from build123d import *

# Parameters (mm, degrees)
BOSS_EXTRUDE1_DEPTH = 12.7
SKETCH2_W           = 4.3815
SKETCH2_H           = 12.607430492
CUT_EXTRUDE1_DEPTH  = 496.623170669
SKETCH3_R           = 5.08
BOSS_EXTRUDE2_DEPTH = 12.7


with BuildPart() as part:
    # Sketch1 → Boss-Extrude1 (new body)
    with BuildSketch(Plane.XY):
        Polygon((0, 0), (0, 6.35), (4.3815, 12.607430492), (5.1435, 12.607430492), (9.525, 6.35), (13.9065, 12.607430492), (14.6685, 12.607430492), (19.05, 6.35), (23.4315, 12.607430492), (24.1935, 12.607430492), (28.575, 6.35), (32.9565, 12.607430492), (33.7185, 12.607430492), (38.1, 6.35), (42.4815, 12.607430492), (43.2435, 12.607430492), (47.625, 6.35), (52.0065, 12.607430492), (52.7685, 12.607430492), (57.15, 6.35), (61.5315, 12.607430492), (62.2935, 12.607430492), (66.675, 6.35), (71.0565, 12.607430492), (71.8185, 12.607430492), (76.2, 6.35), (80.5815, 12.607430492), (81.3435, 12.607430492), (85.725, 6.35), (90.1065, 12.607430492), (90.8685, 12.607430492), (95.25, 6.35), (99.6315, 12.607430492), (100.3935, 12.607430492), (104.775, 6.35), (109.1565, 12.607430492), (109.9185, 12.607430492), (114.3, 6.35), (118.6815, 12.607430492), (119.4435, 12.607430492), (123.825, 6.35), (128.2065, 12.607430492), (128.9685, 12.607430492), (133.35, 6.35), (137.7315, 12.607430492), (138.4935, 12.607430492), (142.875, 6.35), (147.2565, 12.607430492), (148.0185, 12.607430492), (152.4, 6.35), (156.7815, 12.607430492), (157.5435, 12.607430492), (161.925, 6.35), (166.3065, 12.607430492), (167.0685, 12.607430492), (171.45, 6.35), (175.8315, 12.607430492), (176.5935, 12.607430492), (180.975, 6.35), (185.3565, 12.607430492), (186.1185, 12.607430492), (190.5, 6.35), (194.8815, 12.607430492), (195.6435, 12.607430492), (200.025, 6.35), (204.4065, 12.607430492), (205.1685, 12.607430492), (209.55, 6.35), (213.9315, 12.607430492), (214.6935, 12.607430492), (219.075, 6.35), (223.4565, 12.607430492), (224.2185, 12.607430492), (228.6, 6.35), (232.9815, 12.607430492), (233.7435, 12.607430492), (238.125, 6.35), (242.5065, 12.607430492), (243.2685, 12.607430492), (247.65, 6.35), (252.0315, 12.607430492), (252.7935, 12.607430492), (257.175, 6.35), (261.5565, 12.607430492), (262.3185, 12.607430492), (266.7, 6.35), (271.0815, 12.607430492), (271.8435, 12.607430492), (276.225, 6.35), (280.6065, 12.607430492), (281.3685, 12.607430492), (285.75, 6.35), (290.1315, 12.607430492), (290.8935, 12.607430492), (295.275, 6.35), (299.6565, 12.607430492), (300.4185, 12.607430492), (304.8, 6.35), (309.1815, 12.607430492), (309.9435, 12.607430492), (314.325, 6.35), (318.7065, 12.607430492), (319.4685, 12.607430492), (323.85, 6.35), (328.2315, 12.607430492), (328.9935, 12.607430492), (333.375, 6.35), (337.7565, 12.607430492), (338.5185, 12.607430492), (342.9, 6.35), (347.2815, 12.607430492), (348.0435, 12.607430492), (352.425, 6.35), (356.8065, 12.607430492), (357.5685, 12.607430492), (361.95, 6.35), (366.3315, 12.607430492), (367.0935, 12.607430492), (371.475, 6.35), (375.8565, 12.607430492), (376.6185, 12.607430492), (381, 6.35), (385.3815, 12.607430492), (386.1435, 12.607430492), (390.525, 6.35), (394.9065, 12.607430492), (395.6685, 12.607430492), (400.05, 6.35), (404.4315, 12.607430492), (405.1935, 12.607430492), (409.575, 6.35), (413.9565, 12.607430492), (414.7185, 12.607430492), (419.1, 6.35), (423.4815, 12.607430492), (424.2435, 12.607430492), (428.625, 6.35), (433.0065, 12.607430492), (433.7685, 12.607430492), (438.15, 6.35), (442.5315, 12.607430492), (443.2935, 12.607430492), (447.675, 6.35), (452.0565, 12.607430492), (452.8185, 12.607430492), (457.2, 6.35), (461.5815, 12.607430492), (462.3435, 12.607430492), (466.725, 6.35), (471.1065, 12.607430492), (471.8685, 12.607430492), (476.25, 6.35), (480.6315, 12.607430492), (481.3935, 12.607430492), (485.775, 6.35), (490.1565, 12.607430492), (490.9185, 12.607430492), (495.3, 6.35), (495.3, 0), align=None)
    extrude(amount=BOSS_EXTRUDE1_DEPTH)

    # Sketch2 → Cut-Extrude1 (cut, through all)
    with BuildSketch(Plane.XY.offset(12.7)):
        with Locations((493.10925, 6.303715246)):
            Rectangle(SKETCH2_W, SKETCH2_H)
    extrude(amount=-CUT_EXTRUDE1_DEPTH, mode=Mode.SUBTRACT)

    # Sketch3 → Boss-Extrude2 (add)
    with BuildSketch(Plane(origin=(490.9185, 0, 0), x_dir=(0, 0, -1), z_dir=(1, 0, 0))):
        with Locations(Location((-6.35, 6.303715246, 0), (0, 0, 180))):
            Circle(SKETCH3_R)
    extrude(amount=BOSS_EXTRUDE2_DEPTH)


solid = part.part
Check sheet for the modelled part. Datum: model origin and axes. Units: mm. A direction names the side the tool comes from. Round coordinates to 2 decimals unless told otherwise and drop trailing zeros.
1. Scan lines: probe 1 along Y at (x, z) = (242.5, 1.5); probe 2 along X at (y, z) = (1.75, 2.5); probe 3 along Y at (x, z) = (369, 3.75). Record each from-to range of solid material in increasing order.
2. Sectioned sample at A-A on y = 8.5. Give the number of separate pieces and of enclosed holes in the cut face, and give its area (3 significant figures).
3. Set-up check for faces 1 (the cylindrical face through (497.18, 10.811, 8.694)), 2 (the flat face through (249, 5, 12.7)): record each of +Z, -Z, +X, -X, +Y, -Y from which the full face is reachable in a straight line by a thin tool's end or side.
4. Gauge pin test, flat ends, axial feed: pin 1 Ø1 at (x, y) = (106, 4) entering from -Z; pin 2 Ø1.5 at (x, z) = (263.5, 5.5) entering from +Y; pin 3 Ø3 at (y, z) = (8.5, 5.5) entering from -X. Record the tip position at first contact, or that the pin passes through.
Recorded:
1. probe 1: y = 0 to 12.6
1. probe 2: x = 0 to 490.92
1. probe 3: y = 0 to 9.88
2. separate pieces: 52
2. enclosed holes: 0
2. area: 4,380 mm2
3. face 1: +X
3. face 2: +Z, +X, -X, +Y, -Y
4. pin 1: stops at z = 0
4. pin 2: stops at y = 11.99
4. pin 3: stops at x = 0.46
